Drawing for the job (mm, zero at the part's lowest x, y, z). Coordinates: 2 decimals unless noted, no trailing zeros. Write each loop counter-clockwise with the first axis right and the second up, starting at its lowest first coordinate (ties: lowest second). Pieces come first, ordered by that corner, then holes. Notation, with made-up numbers: M -1.5,38.25 L 2.5,38.25 A15 ccw 2.5,54.25 Z; hole C 78,69 d3. An arc over 180 degrees is marked long. Put each result on its own line as item: value. Start each with the question number.
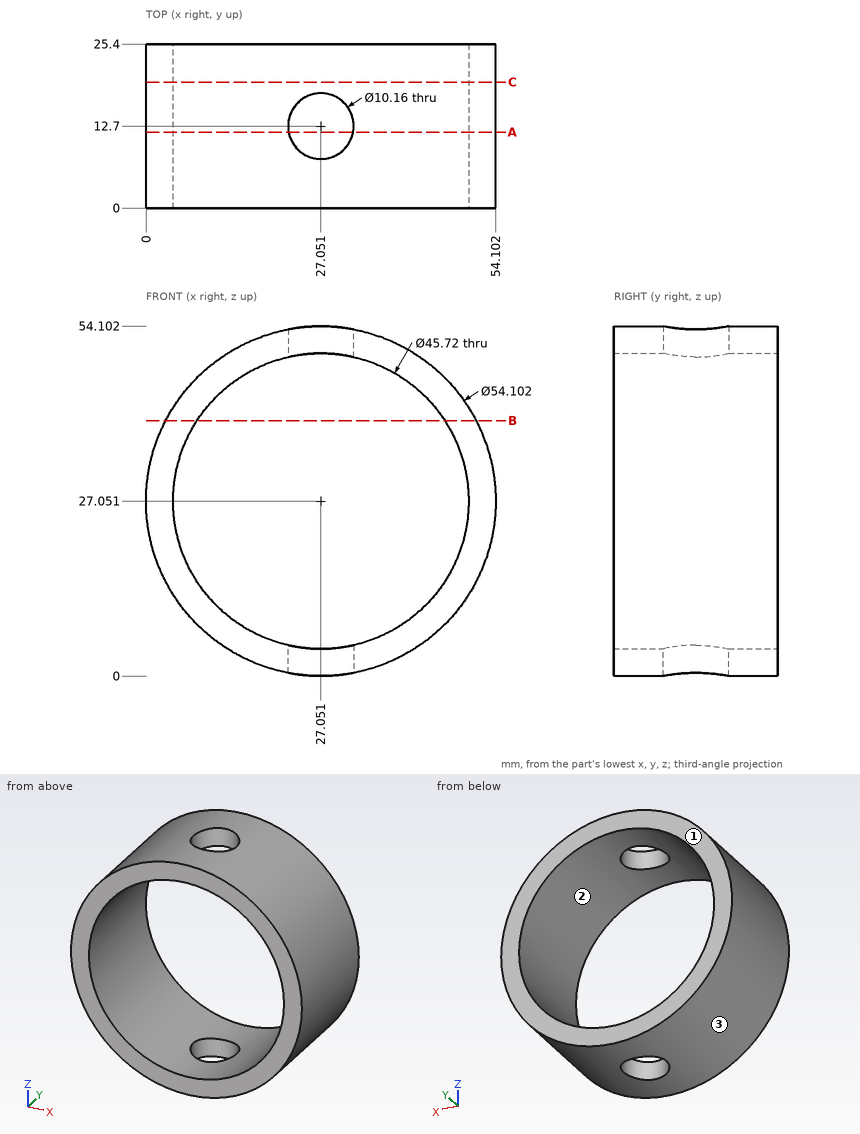
(1) Slice it at C-C, the plane y = 19.5. Write the cut outline in (x, z), then the cut area to 3 significant figures.
(2) Drill centre lines: line 1 (X direction, y = 20.25, z = 27.5); line 2 (X direction, y = 4.5, z = 6); line 3 (Z direction, x = 43, y = 2). Where is each one in solid material? Low to high. Write a range as [from, to].
(3) Slice it at A-A, the plane y = 11.75. Write the cut outline in (x, z), then the cut area to 3 significant figures.
(4) Two-plate mould, pull along X, no slides. Class the marked faces 1, 2 and 3: +X half, -X half, draft (parallel to the pull), parting line (faces both ways), or undercut.
(5) Slice it at B-B, the plane z = 39.5. Write the cut outline in (x, y).
(6) Drop flat-ended pins along their axis: pin 1 (2 mm diameter, centred on x = 36, y = 12, fed in from -Z); pin 2 (6 mm diameter, centred on y = 11, z = 14, fed in from +X); pin 3 (1.5 mm diameter, centred on x = 35, y = 17, fed in from +Z); pin 4 (9 mm diameter, centred on x = 27.051, y = 12.7, fed in from -Z). Give the stop position or say it passes through.
Result set:
1. outline: C 27.05,27.05 d54.1; hole C 27.05,27.05 d45.72
1. area: 657 mm^2
2. line 1: x = [0, 4.2], [49.91, 54.1]
2. line 2: x = [10.06, 18.14], [35.96, 44.04]
2. line 3: z = [5.2, 10.67], [43.43, 48.9]
3. outline: M 22.06,0.46 L 22.06,4.74 A22.86 cw 22.06,49.36 L 22.06,53.64 A27.05 ccw Z; M 32.04,0.46 A27.05 ccw 32.04,53.64 L 32.04,49.36 A22.86 cw 32.04,4.74 Z
3. area: 573 mm^2
4. face 1: draft
4. face 2: undercut
4. face 3: parting line
5. outline: M 3.03,0 L 7.88,0 L 7.88,25.4 L 3.03,25.4 Z; M 46.22,0 L 51.07,0 L 51.07,25.4 L 46.22,25.4 Z
6. pin 1: stops at z = 1.19
6. pin 2: stops at x = 52.17
6. pin 3: stops at z = 53.13
6. pin 4: passes through
